For this review, take the finished solid that the model builds, in its own axes (mm). Face numbers are marked on the shaded views. Round coordinates to 2 decimals unless told otherwise and drop trailing zeros. Write each loop counter-clockwise with the first axis right and the second up, starting at its lowest first coordinate (ties: lowest second). Pieces come first, ordered by that corner, then holes. Notation, with made-up numbers: M -20.5,36.5 L 31.5,36.5 A18 cw 31.5,65.5 Z; hole C 20,53.25 d3. An arc over 180 degrees is marked long. Use one line per item in the form item = value. Start each with the question number.
Item 1: Add section A-A (z = 0). State the section outline as (x, y) points, and give its area (3 significant figures).
Item 2: Add section B-B (x = 0). State the section outline as (y, z) points, and give its area (3 significant figures).
Item 3: Add section C-C (z = 49.5). State the section outline as (x, y) points, and give its area (3 significant figures).
Item 4: Add section D-D (x = 27). State the section outline as (y, z) points.
Item 5: For P1, Ø1.5, axis at x = -87.5, y = 1, coming from the +Z side; P2, Ø1.5, axis at x = 68.5, z = -4, coming from the -Y side, all flat-tipped, find the tip position at first contact; note any pin that passes through.
Item 6: Draft analysis for pull direction Y (two halves, no side actions). For the marked faces 1 and 2, state which applies: released by +Y, released by -Y, zero draft, split by the parting line, or undercut.
Item 7: For line 1 (Z direction, x = 44.5, y = 1.5); line 2 (Z direction, x = 0, y = 1.6); line 3 (X direction, y = 2.3, z = 46), list the stretches that pass through material, from the lowest coordinate up. Write a range as [from, to].
Autodesk Inventor part; units mm, degrees
ref_plane "YZ Plane" through (0, 0, 0) normal (1, 0, 0) x (0, 1, 0)
ref_plane "XZ Plane" through (0, 0, 0) normal (0, 1, 0) x (-1, 0, 0)
ref_plane "XY Plane" through (0, 0, 0) normal (0, 0, 1) x (1, 0, 0)
sketch "Sketch2" plane through (0, 0, 0) normal (0, 1, 0) x (-1, 0, 0)
  line L0 (90, -53) -> (84, -53)
  line L1 (84, -53) -> (84, -43)
  line L2 (84, -43) -> (90, -43)
  line L3 (-90, -53) -> (-84, -53)
  line L4 (-84, -53) -> (-84, -43)
  line L5 (-84, -43) -> (-90, -43)
  line L6 (70, -18) -> (60, -18)
  line L7 (60, -18) -> (60, -15)
  line L8 (60, -15) -> (70, -15)
  line L9 (70, -15) -> (70, -18)
  line L10 (-70, -18) -> (-60, -18)
  line L11 (-60, -18) -> (-60, -15)
  line L12 (-60, -15) -> (-70, -15)
  line L13 (-70, -15) -> (-70, -18)
  circle A0 centre (0, 0) radius 38.05
  line L14 (46.5, -15) -> (43.5, -15)
  line L15 (43.5, -15) -> (43.5, -5)
  line L16 (43.5, -5) -> (46.5, -5)
  line L17 (46.5, -5) -> (46.5, -15)
  line L18 (-46.5, -15) -> (-43.5, -15)
  line L19 (-43.5, -15) -> (-43.5, -5)
  line L20 (-43.5, -5) -> (-46.5, -5)
  line L21 (-46.5, -5) -> (-46.5, -15)
  line L22 (43.5, 57) -> (43.5, 47)
  line L23 (43.5, 47) -> (46.5, 47)
  line L24 (46.5, 47) -> (46.5, 57)
  line L25 (-46.5, 47) -> (-43.5, 47)
  line L26 (-43.5, 47) -> (-43.5, 57)
  line L27 (-46.5, 57) -> (-46.5, 47)
  line L28 (-85, 85) -> (85, 85)
  arc A1 (-85, 85) -> (-90, 80) centre (-85, 80) ccw
  arc A2 (90, 80) -> (85, 85) centre (85, 80) ccw
  line L29 (46.5, 57) -> (43.5, 57)
  line L30 (-43.5, 57) -> (-46.5, 57)
  line L31 (30, 57) -> (20, 57)
  line L32 (20, 57) -> (20, 60)
  line L33 (20, 60) -> (30, 60)
  line L34 (30, 60) -> (30, 57)
  line L35 (-20, 57) -> (-30, 57)
  line L36 (-30, 57) -> (-30, 60)
  line L37 (-30, 60) -> (-20, 60)
  line L38 (-20, 60) -> (-20, 57)
  line L39 (3, 70) -> (-3, 70)
  line L40 (-3, 70) -> (-3, 80)
  line L41 (-3, 80) -> (3, 80)
  line L42 (3, 80) -> (3, 70)
  line L43 (3, 45) -> (-3, 45)
  line L44 (-3, 45) -> (-3, 55)
  line L45 (-3, 55) -> (3, 55)
  line L46 (3, 55) -> (3, 45)
  line L47 (-90, -43) -> (-90, 80)
  line L48 (90, 80) -> (90, -43)
  line L49 (90, -53) -> (90, -65)
  line L50 (-90, -53) -> (-90, -65)
  line L51 (90, -65) -> (-90, -65)
  point P0 (-91.6845, 9.0823)
  point P1 (90, 85)
  dimension "d21" = 6
  dimension "d22" = 10
  dimension "d25" = 6
  dimension "d26" = 10
  dimension "d31" = 3
  dimension "d32" = 10
  dimension "d35" = 3
  dimension "d36" = 10
  dimension "d39" = 25
  dimension "d40" = 25
  dimension "d43" = 76.1
  dimension "d52" = 3
  dimension "d53" = 10
  dimension "d54" = 10
  dimension "d55" = 3
  dimension "d58" = 10
  dimension "d59" = 3
  dimension "d62" = 3
  dimension "d65" = 180
  dimension "d66" = 150
  dimension "d90" = 90
  dimension "d91" = 90
  dimension "d103" = 10
  dimension "d104" = 10
  dimension "d108" = 3
  dimension "d109" = 10
  dimension "d110" = 20
  dimension "d111" = 3
  dimension "d112" = 10
  dimension "d113" = 20
  dimension "d114" = 5
  dimension "d115" = 10
  dimension "d116" = 6
  dimension "d117" = 3
  dimension "d118" = 10
  dimension "d119" = 6
  dimension "d120" = 15
  dimension "d121" = 3
extrude "Extrusion6" add sketch "Sketch2" along normal blind 3
properties part number "OpenROV 2_2a Top"
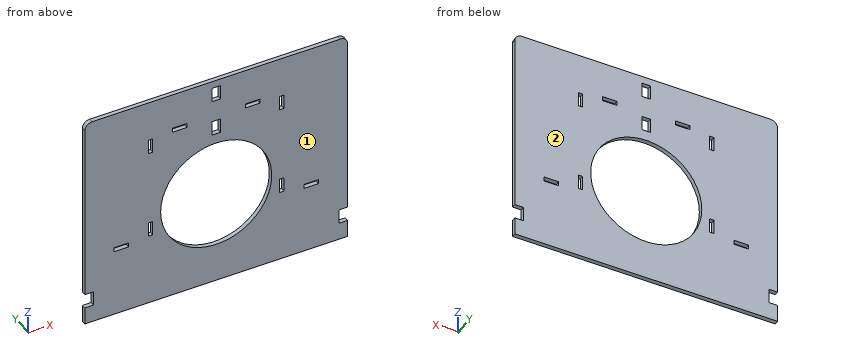
Calculated:
q1.outline = M -90,0 L -38.05,0 L -38.05,3 L -90,3 Z; M 38.05,0 L 90,0 L 90,3 L 38.05,3 Z
q1.area = 312 mm^2
q2.outline = M 0,-65 L 3,-65 L 3,-38.05 L 0,-38.05 Z; M 0,38.05 L 3,38.05 L 3,45 L 0,45 Z; M 0,55 L 3,55 L 3,70 L 0,70 Z; M 0,80 L 3,80 L 3,85 L 0,85 Z
q2.area = 162 mm^2
q3.outline = M -90,0 L -46.5,0 L -46.5,3 L -90,3 Z; M -43.5,0 L -3,0 L -3,3 L -43.5,3 Z; M 3,0 L 43.5,0 L 43.5,3 L 3,3 Z; M 46.5,0 L 90,0 L 90,3 L 46.5,3 Z
q3.area = 504 mm^2
q4.outline = M 0,-65 L 3,-65 L 3,-26.81 L 0,-26.81 Z; M 0,26.81 L 3,26.81 L 3,57 L 0,57 Z; M 0,60 L 3,60 L 3,85 L 0,85 Z
q5.P1 = 84.68
q5.P2 = 0
q6.face_1 = released by -Y
q6.face_2 = released by +Y
q7.line_1 = [-65, -15], [-5, 47], [57, 85]
q7.line_2 = [-65, -38.05], [38.05, 45], [55, 70], [80, 85]
q7.line_3 = [-90, -3], [3, 90]
